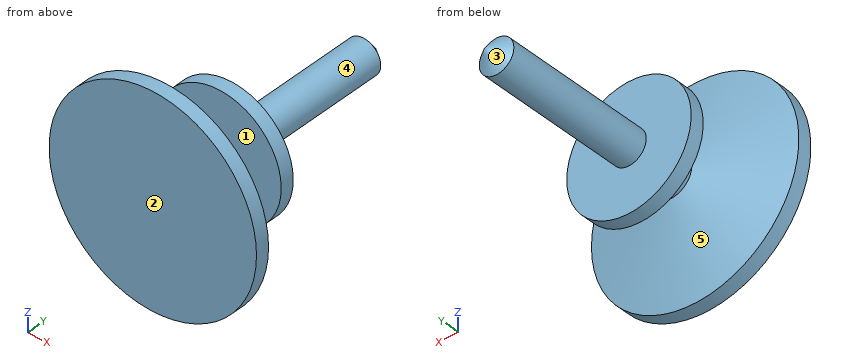
Autodesk Inventor part; units mm, degrees
ref_plane "YZ Plane" through (0, 0, 0) normal (1, 0, 0) x (0, 1, 0)
ref_plane "XZ Plane" through (0, 0, 0) normal (0, 1, 0) x (-1, 0, 0)
ref_plane "XY Plane" through (0, 0, 0) normal (0, 0, 1) x (1, 0, 0)
sketch "Skizze3" plane through (0, 0, 0) normal (0, 0, 1) x (1, 0, 0)
  line L0 (0, 0) -> (15, 0)
  line L1 (15, 0) -> (15, 2)
  line L2 (15, 2) -> (3, 6)
  line L3 (3, 6) -> (3, 11)
  line L4 (3, 11) -> (9, 11)
  line L5 (9, 11) -> (9, 13)
  line L6 (9, 13) -> (2.5, 13)
  line L7 (2.5, 13) -> (2.5, 35)
  line L8 (2.5, 35) -> (0, 37)
  line L9 (0, -1.3947) -> (0, 46.3421)
  dimension "d4" = 18
  dimension "d5" = 6
  dimension "d6" = 2
  dimension "d7" = 5
  dimension "d8" = 2
  dimension "d9" = 6
  dimension "d11" = 5
  dimension "d12" = 30
  dimension "d13" = 35
  dimension "d14" = 2
revolve "Umdrehung1" add sketch "Skizze3" angle 360 about axis through (0, -1.3947, 0) along (0, 1, 0)
thread "Gewinde1"
properties part number "BT002_trajan20_22" material "Kunststoff, undurchsichtig Schwarz"
The model under review builds one solid part; all positions refer to its coordinate system, in mm. Face numbers are marked on the shaded views. A direction names the side the tool comes from. Round coordinates to 2 decimals unless told otherwise and drop trailing zeros. Order: outer loops, then holes, each group sorted by start corner. A loop starts at its lowest first (then second) coordinate and runs counter-clockwise, first axis right, second up. Notation, with made-up numbers: (-40, 34) -> (-15, 34) arc R19 ccw to (-15, 69) -> close; hole circle Ø1 at (-29.75, 77). An arc over 180 degrees is marked (long way). Use CSV: the item, a comma, the result in double quotes. Start each with the question number.
(1) Insertion check: pin 1 (5 mm diameter, centred on x = -5, y = 12.5, fed in from +Z); pin 2 (1.5 mm diameter, centred on x = 6.5, z = -6, fed in from +Y); pin 3 (6 mm diameter, centred on x = -5.5, y = 11.5, fed in from -Z). Each pin has a flat end and moves straight along its axis. Give the tip position at first contact, or say it passes through.
(2) Consider section A-A on y = 15.5. Write out the cut boundary in (x, z).
(3) Tool access review of the marked faces 4 and 5: name each direction out of +Z, -Z, +X, -X, +Y, -Y from which nothing blocks a thin tool from reaching the whole face with its end or side.
(4) Mouldability with a two-part tool opening along Y and no side actions: class the marked faces 1, 2 and 3 as pulls with the +Y half, pulls with the -Y half, needs draft (parallel to the pull), parting line crosses it, or undercut.
(5) Wall thickness on probe 1 along Y at (x, z) = (-2.5, -2.5); probe 2 along Y at (x, z) = (2.5, 7.75); probe 3 along X at (y, z) = (17, -2): over which ranges is each line inside the solid? List them lowest first. Write a range as from..to.
(6) Consider section B-B on y = 8. Write out the cut boundary in (x, z), and give its area (3 significant figures).
Responses:
1,pin 1,"z = 8.65"
1,pin 2,"y = 13"
1,pin 3,"z = -8.65"
2,outline,"circle Ø5 at (0, 0)"
3,face 4,"+Y"
3,face 5,"none"
4,face 1,"undercut"
4,face 2,"pulls with the -Y half"
4,face 3,"pulls with the +Y half"
5,probe 1,"0..5.82, 11..13"
5,probe 2,"0..4.29, 11..13"
5,probe 3,"-1.5..1.5"
6,outline,"circle Ø6 at (0, 0)"
6,area,"28.3 mm²"
